Answer from the drawing. Dimensions are ordinates in mm from the lowest x, y and z of the part. A direction names the side the tool comes from. Round coordinates to 2 decimals unless told otherwise and drop trailing zeros. Order: outer loops, then holes, each group sorted by start corner. A loop starts at its lowest first (then second) coordinate and runs counter-clockwise, first axis right, second up. Notation, with made-up numbers: (26.5, -4.5) -> (58.5, -4.5) arc R32 cw to (58.5, 26.5) -> close; hole circle Ø8 at (-32.5, 67). An arc over 180 degrees is marked (long way). Use a Markdown table: item, result. Add a question column.
Item 1: A cutting plane is placed at A-A, the plane y = 12.5. Determine the outline of the cut face in (x, z).
Item 2: Flat-ended cylindrical pins translate along their axes: P1, Ø4, axis at x = 8.5, z = 4, coming from the +Y side; P2, Ø6, axis at x = 12.5, y = 12.5, coming from the -Z side; P3, Ø3, axis at y = 17, z = 2, coming from the +X side; P4, Ø15, axis at x = 12.5, y = 12.5, coming from the -Z side. Find the tip coordinate at first contact, or state that the pin passes through.
Item 3: A tool of negligible diameter and unlimited length cuts with its end or side. For the marked faces 4 and 5, from which of +Z, -Z, +X, -X, +Y, -Y can it reach the whole face along a straight path? Write none if from no direction.
Item 4: A cutting plane is placed at C-C, the plane z = 5. Determine the outline of the cut face in (x, y), plus the area to 3 significant figures.
Item 5: For a pull along Y with two mould halves and no side action, classify the marked faces 1, 2 and 3 as +Y half, -Y half, draft (parallel to the pull), parting line (faces both ways), or undercut.
Item 6: Find the intervals of material crossed by L1, parallel to Y at x = 12.5, z = 1.85; L2, parallel to Y at x = 18, z = 2.75; L3, parallel to Z at x = 7, y = 8.5, in increasing order. Write a range as [from, to].
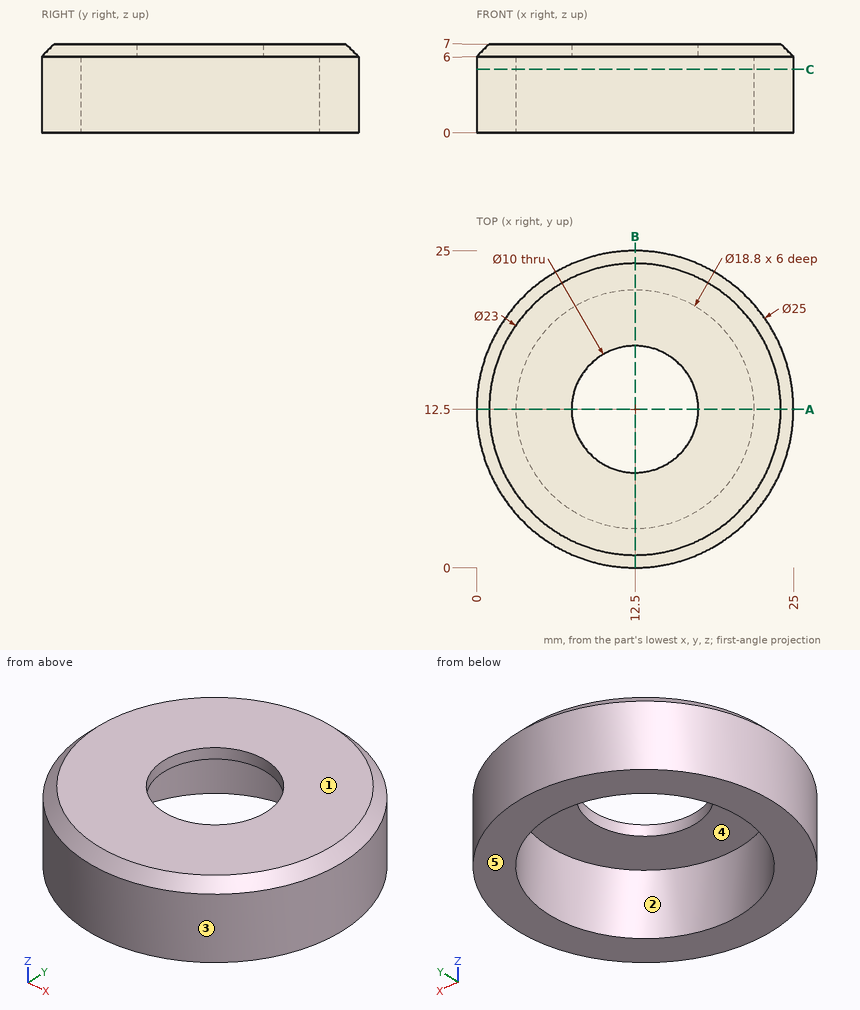
Reported:
| question | item | result |
|---|---|---|
| 1 | outline | (0, 0) -> (3.1, 0) -> (3.1, 6) -> (7.5, 6) -> (7.5, 7) -> (1, 7) -> (0, 6) -> close; (17.5, 6) -> (21.9, 6) -> (21.9, 0) -> (25, 0) -> (25, 6) -> (24, 7) -> (17.5, 7) -> close |
| 2 | P1 | y = 24.84 |
| 2 | P2 | through |
| 2 | P3 | x = 24.63 |
| 2 | P4 | z = 6 |
| 3 | face 4 | -Z |
| 3 | face 5 | -Z, +X, -X, +Y, -Y |
| 4 | outline | circle Ø25 at (12.5, 12.5); hole circle Ø18.8 at (12.5, 12.5) |
| 4 | area | 213 mm² |
| 5 | face 1 | draft |
| 5 | face 2 | undercut |
| 5 | face 3 | parting line |
| 6 | L1 | [0, 3.1], [21.9, 25] |
| 6 | L2 | [1.28, 4.88], [20.12, 23.72] |
| 6 | L3 | [6, 7] |
